Geometry: see drawing. Coordinates: mm, zero at the bounding-box minimum. A direction names the side the tool comes from. Round coordinates to 2 decimals unless told otherwise and drop trailing zeros. Order: outer loops, then holes, each group sorted by start corner. A loop starts at its lowest first (then second) coordinate and runs counter-clockwise, first axis right, second up. Notation, with made-up numbers: (19, -4) -> (44, -4) arc R34 ccw to (44, 28) -> close; hole circle Ø3 at (5.25, 71). An arc over 180 degrees is marked (long way). One line per item, written item: value. Start each with the question number.
1) Section B-B (x = 9.65). Return the cut outline in (y, z), and give its area (3 significant figures).
2) Pin query (flat end, axial travel): P1, Ø2, axis at y = 1, z = 4, coming from the -X side; P2, Ø1.6, axis at x = 15, y = 1.5, coming from the -Z side; P3, Ø1.5, axis at x = 12.5, y = 7.5, coming from the -Z side; P4, Ø10, axis at x = 11.5, y = 17.5, coming from the +Z side. Return the tip coordinate at first contact, or that it passes through.
3) Section A-A (z = 9.65). Return the cut outline in (x, y), and give its area (3 significant figures).
4) Section D-D (x = 3). State how many separate pieces and enclosed holes the cut face has, and give its area (3 significant figures).
5) Section C-C (y = 6.5). Return the cut outline in (x, z).
6) Ray query, L1, parallel to X at y = 1.3, z = 9.65; L2, parallel to X at y = 24.5, z = 9.5; L3, parallel to Y at x = 4.75, z = 7. Return the intervals inside material, ascending.
7) Mould query, pull axis Y, two halves, no side actions, for the marked faces 1, 2 and 3. Classes: pulls with the +Y half, pulls with the -Y half, needs draft (parallel to the pull), parting line crosses it, or undercut.
8) Reachability of the marked faces 4, 5, 6 and 7 from +Z, -Z, +X, -X, +Y, -Y: full face, straight path, thin tool, end or side. Return the list, or none.
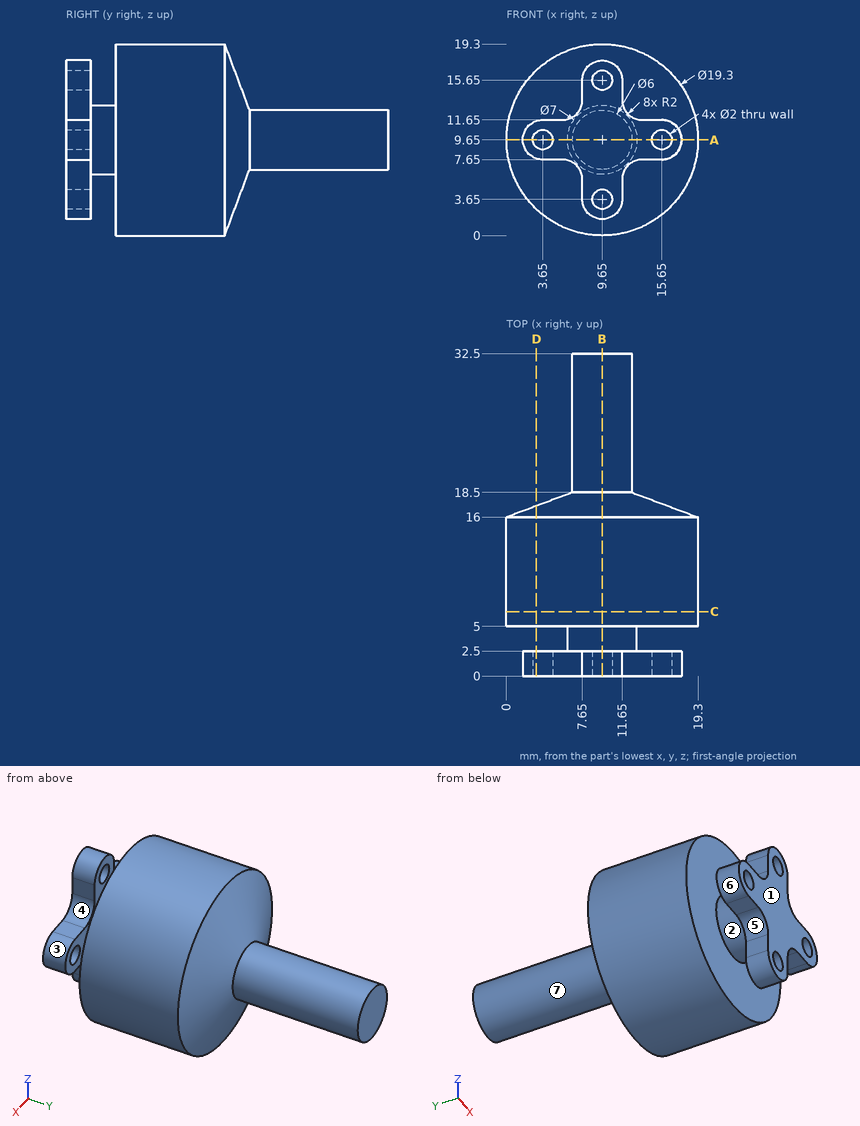
Findings:
1. outline: (0, 1.65) -> (2.5, 1.65) -> (2.5, 2.65) -> (0, 2.65) -> close; (0, 4.65) -> (2.5, 4.65) -> (2.5, 6.15) -> (5, 6.15) -> (5, 0) -> (16, 0) -> (18.5, 6.65) -> (32.5, 6.65) -> (32.5, 12.65) -> (18.5, 12.65) -> (16, 19.3) -> (5, 19.3) -> (5, 13.15) -> (2.5, 13.15) -> (2.5, 14.65) -> (0, 14.65) -> close; (0, 16.65) -> (2.5, 16.65) -> (2.5, 17.65) -> (0, 17.65) -> close
1. area: 375 mm2
2. P1: x = 7.65
2. P2: z = 7.65
2. P3: z = 0.23
2. P4: z = 19.3
3. outline: (0, 5) -> (6.15, 5) -> (6.15, 2.5) -> (4.65, 2.5) -> (4.65, 0) -> (14.65, 0) -> (14.65, 2.5) -> (13.15, 2.5) -> (13.15, 5) -> (19.3, 5) -> (19.3, 16) -> (12.65, 18.5) -> (12.65, 32.5) -> (6.65, 32.5) -> (6.65, 18.5) -> (0, 16) -> close; (1.65, 0) -> (2.65, 0) -> (2.65, 2.5) -> (1.65, 2.5) -> close; (16.65, 0) -> (17.65, 0) -> (17.65, 2.5) -> (16.65, 2.5) -> close
3. area: 375 mm2
4. separate pieces: 3
4. enclosed holes: 0
4. area: 170 mm2
5. outline: circle Ø19.3 at (9.65, 9.65)
6. L1: 1.65 to 2.65, 4.65 to 14.65, 16.65 to 17.65
6. L2: 6.65 to 12.65
6. L3: 5 to 17.53
7. face 1: pulls with the -Y half
7. face 2: undercut
7. face 3: needs draft
8. face 4: +Z, +X, -Y
8. face 5: -Z, -X, -Y
8. face 6: -X, -Y
8. face 7: +Y
